Autodesk Inventor part; units mm, degrees
ref_plane "YZ Plane" through (0, 0, 0) normal (1, 0, 0) x (0, 1, 0)
ref_plane "XZ Plane" through (0, 0, 0) normal (0, 1, 0) x (-1, 0, 0)
ref_plane "XY Plane" through (0, 0, 0) normal (0, 0, 1) x (1, 0, 0)
sketch "Sketch2" plane through (0, 0, 0) normal (0, 1, 0) x (-1, 0, 0)
  circle A0 centre (0, 0) radius 9
  dimension "d2" = 18
extrude "Extrusion2" add sketch "Sketch2" along normal blind 60
hole "Hole1" at (0, 0, 0) direction (0, 1, 0) diameter 8.376 depth 25 tip angle 118 countersink diameter 10 countersink angle 118
sketch "Sketch3" plane through (0, 60, 0) normal (0, 1, 0) x (1, 0, 0)
  point P0 (0, 0)
  point P1 (0, 0)
hole "Hole2" at (0, 60, 0) direction (0, -1, 0) diameter 14 depth 15 tip angle 118
sketch "Sketch4" plane through (0, 0, 0) normal (0, 0, 1) x (1, 0, 0)
  circle A0 centre (0, 53) radius 4
  line L0 (9, 60) -> (-9, 60)
  point P0 (0, 0)
  point P1 (0, 60)
  dimension "d20" = 8
  dimension "d21" = 7
extrude "Extrusion3" cut sketch "Sketch4" along normal through all both and the other way through all
chamfer "Chamfer3" distance 0.5 angle 45 1 edges at (0, 60, -7)
sketch "Sketch6" plane through (0, 60, 0) normal (0, 1, 0) x (1, 0, 0)
  circle A0 centre (0, 0) radius 9
  line L0 (-9, 0) -> (9, 0)
  line L1 (9, 0) -> (9, 9)
  line L2 (9, 9) -> (-9, 9)
  line L3 (-9, 9) -> (-9, 0)
  dimension "d38" = 9
  dimension "d39" = 18
extrude "Extrusion5" [suppressed]
properties part number "RS-STT-103" material "11 110 (1.0721)"
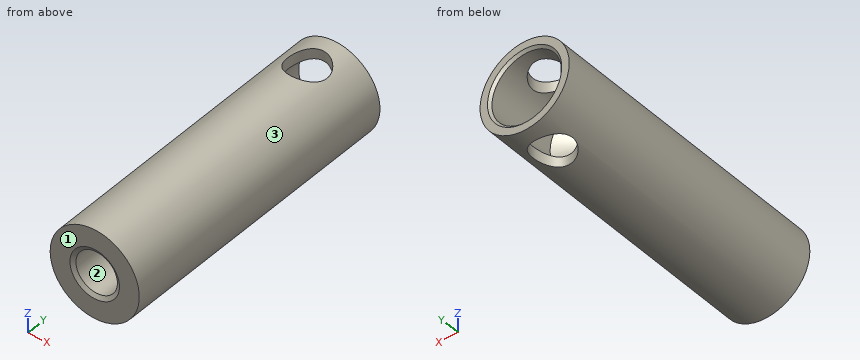
Could you check a few things on this model? Use its own coordinates, in mm. Face numbers are marked on the shaded views. Coordinates: 2 decimals unless noted, no trailing zeros. Loops run counter-clockwise (first coordinate to the right, second up) from the corner with the lowest first, then second, coordinate; pieces in that order, holes last.
1) Will these pins go through, and if not, where does the flat tip stop? pin 1 Ø6.5 at (x, z) = (0, 0) entering from -Y; pin 2 Ø1 at (y, z) = (37, -2.5) entering from -X; pin 3 Ø1 at (x, z) = (0.5, -4.5) entering from +Y.
Reported:
pin 1: stops at y = 25.56
pin 2: stops at x = -8.77
pin 3: stops at y = 43.81
2) Thinking about a two-plate mould opening in X: for the marked faces 1, 2 and 3, which applies, released by +X, released by -X, zero draft, split by the parting line, or undercut?
Reported:
face 1: zero draft
face 2: undercut
face 3: split by the parting line
3) Imagine slicing it at D-D (y = 34.5). List the corners of the cut face in (x, z) for me, and give its area (3 significant figures).
Reported:
outline: circle Ø18 at (0, 0)
area: 254 mm2
4) Imagine slicing it at A-A (y = 50). List the corners of the cut face in (x, z) for me, and give its area (3 significant figures).
Reported:
outline: (-2.65, -8.6) - (-2.65, -6.48) arc R7 cw to (-2.65, 6.48) - (-2.65, 8.6) arc R9 ccw to start; (2.65, -8.6) arc R9 ccw to (2.65, 8.6) - (2.65, 6.48) arc R7 cw to (2.65, -6.48) - close
area: 79.0 mm2
5) Imagine slicing it at B-B (x = -2.5). State how many separate pieces and enclosed holes the cut face has, and give its area (3 significant figures).
Reported:
separate pieces: 3
enclosed holes: 0
area: 621 mm2
6) Imagine slicing it at C-C (y = 17.5). List the corners of the cut face in (x, z) for me, and give its area (3 significant figures).
Reported:
outline: circle Ø18 at (0, 0); hole circle Ø8.38 at (0, 0)
area: 199 mm2
7) Please list where these lines run through material, in increasing order: line 1 along Y through (x, z) = (0, 8); line 2 along X through (y, z) = (53, -7.2); line 3 along X through (y, z) = (10.5, 1).
Reported:
line 1: y = 0 to 49, 57 to 60
line 2: x = -5.4 to -4, 4 to 5.4
line 3: x = -8.94 to -4.07, 4.07 to 8.94
